```python
from build123d import *

# Parameters (mm, degrees)
SKETCH1_R             = 1.4000000000000001
BOSS_EXTRUDE1_DEPTH   = 8
SKETCH1_R_2           = 1.4000001329680465
BOSS_EXTRUDE1_2_DEPTH = 8
CUT_EXTRUDE1_DEPTH    = 2
BOSS_EXTRUDE2_REACH   = 38.543
FILLET1_R             = 0.3
FILLET2_R             = 0.5
SKETCH4_W             = 3.300000288709998
SKETCH4_H             = 17
BOSS_EXTRUDE3_DEPTH   = 89
FILLET3_R             = 3
FILLET4_R             = 1
FILLET5_R             = 30
FILLET6_R             = 1
FILLET7_R             = 1
SKETCH5_R             = 1.4000008127885915
CUT_EXTRUDE2_DEPTH    = 117.20130403381272


with BuildPart() as part:
    # Sketch1 → Boss-Extrude1 (new body)
    with BuildSketch(Plane.XY):
        Polygon((-3.0301585163921114, 15.386126765608788), (-18.49637259864768, 15.386126765608788), (-25.90000070631504, 14.542589808684392), (-25.90000070631504, 9.120777419209476), (-3.030158516392113, 9.12077741920948), align=None)
        with Locations((-8.999999881867154, 12.49999987202729)):
            Circle(SKETCH1_R, mode=Mode.SUBTRACT)
    extrude(amount=BOSS_EXTRUDE1_DEPTH)


with BuildPart() as body_2:
    # Sketch1 → Boss-Extrude1 2 (new body)
    with BuildSketch(Plane.XY):
        Polygon((-3.0301585163921114, -15.386126765608788), (-3.0301585163921114, -9.12077741920948), (-25.90000070631504, -9.12077741920948), (-25.90000070631504, -14.542589808684392), (-18.496372598647696, -15.386126765608788), align=None)
        with Locations((-8.999999825719202, -12.500000716819214)):
            Circle(SKETCH1_R_2, mode=Mode.SUBTRACT)
    extrude(amount=BOSS_EXTRUDE1_2_DEPTH)


with BuildPart() as cut_extrude1_tool:
    # Sketch2 → Cut-Extrude1 (new body)
    with BuildSketch(Plane.XY.offset(8)):
        Polygon((-5.997778482081098, 12.499999872027288), (-7.498889181974129, 15.099999872027293), (-8.281088680356937, 16.454809144881214), (-9.718911083377371, 16.454809144881214), (-10.501110581760184, 15.099999872027293), (-12.002221281653215, 12.499999872027287), (-10.501110581760186, 9.899999872027289), (-7.498889181974125, 9.899999872027289), align=None)
        Polygon((-7.498889125826173, -9.900000716819214), (-10.501110525612221, -9.900000716819216), (-12.002221225505249, -12.500000716819212), (-10.501110525612223, -15.100000716819206), (-9.468316266504699, -16.88885284735889), (-8.531683384933698, -16.888852847358898), (-7.498889125826177, -15.100000716819206), (-5.997778425933152, -12.500000716819208), align=None)
    extrude(amount=-CUT_EXTRUDE1_DEPTH)


with BuildPart() as part_1:
    add(part.part)

    # Cut-Extrude1: cut by cut_extrude1_tool
    add(cut_extrude1_tool.part, mode=Mode.SUBTRACT)


with BuildPart() as body_2_1:
    add(body_2.part)

    # Cut-Extrude1: cut by cut_extrude1_tool
    add(cut_extrude1_tool.part, mode=Mode.SUBTRACT)

    # Sketch3 → Boss-Extrude2 (add, up to next)
    with BuildSketch(Plane.XZ.offset(-9.12077741920948), mode=Mode.PRIVATE) as boss_extrude2_sk1:
        Polygon((-25.90000070631504, 8), (-25.90000070631504, 2.699999711290002), (-24.255957938355465, 2.6999997112900025), (-12.725226135105776, 8), (-18.496372598647696, 8), align=None)
    boss_extrude2_tool1 = extrude(boss_extrude2_sk1.sketch, amount=BOSS_EXTRUDE2_REACH, mode=Mode.PRIVATE) - body_2_1.part

    add(part_1.part)  # Boss-Extrude2 merges part
    add(boss_extrude2_tool1.solids().sort_by_distance((-21.447611, 9.120777, 6.037334))[0])

    # Fillet1
    fillet1_edges = [body_2_1.edges().sort_by_distance(p)[0] for p in [
        (-10.335915142728517, 15.386126765608788, 7),
        (-7.664084621005797, 15.386126765608788, 7),
        (-7.664084077117004, -15.386126765608788, 7),
        (-10.33591557432139, -15.386126765608788, 7),
    ]]
    fillet(fillet1_edges, radius=FILLET1_R)

    # Fillet2
    fillet2_edges = [body_2_1.edges().sort_by_distance(p)[0] for p in [
        (-12.725226135105776, 0, 8),
    ]]
    fillet(fillet2_edges, radius=FILLET2_R)

    # Sketch4 → Boss-Extrude3 (add)
    with BuildSketch(Plane.ZY.offset(25.90000070631504)):
        with Locations((6.349999855645001, 0)):
            Rectangle(SKETCH4_W, SKETCH4_H)
    extrude(amount=BOSS_EXTRUDE3_DEPTH)

    # Fillet3
    fillet3_edges = [body_2_1.edges().sort_by_distance(p)[0] for p in [
        (-114.90000070631504, 8.5, 6.349999855645001),
        (-114.90000070631504, -8.5, 6.349999855645001),
    ]]
    fillet(fillet3_edges, radius=FILLET3_R)

    # Fillet4
    fillet4_edges = [body_2_1.edges().sort_by_distance(p)[0] for p in [
        (-3.0301585163921114, 15.386126765608788, 4),
        (-3.0301585163921123, 9.12077741920948, 4),
        (-25.90000070631504, 14.542589808684392, 4),
        (-25.90000070631504, 9.120777419209476, 1.349999855645001),
        (-3.0301585163921114, -9.12077741920948, 4),
        (-25.90000070631504, -9.12077741920948, 1.349999855645001),
        (-25.90000070631504, -14.542589808684392, 4),
        (-3.0301585163921114, -15.386126765608788, 4),
    ]]
    fillet(fillet4_edges, radius=FILLET4_R)

    # Fillet5
    fillet5_edges = [body_2_1.edges().sort_by_distance(p)[0] for p in [
        (-18.49637259864768, 15.38612676560879, 4),
        (-18.496372598647696, -15.386126765608788, 4),
    ]]
    fillet(fillet5_edges, radius=FILLET5_R)

    # Fillet6
    fillet6_edges = [body_2_1.edges().sort_by_distance(p)[0] for p in [
        (-14.465079611353577, 9.120777419209478, 0),
        (-22.601074828066285, 14.918454973167087, 0),
        (-3.0301585163921114, 12.253452092409134, 0),
        (-25.90000070631504, 11.885416556829192, 0),
        (-3.323051735205564, 15.093233546795336, 0),
        (-3.3230517352055653, 9.413670638022932, 0),
        (-25.646058085143018, 14.315937356229982, 0),
        (-25.607107487501587, 9.413670638022928, 0),
        (-25.90000070631504, -11.885416556829192, 0),
        (-14.465079611353575, -9.12077741920948, 0),
        (-3.0301585163921114, -12.253452092409134, 0),
        (-10.411503745491025, -15.386126765608788, 0),
        (-3.323051735205564, -9.413670638022932, 0),
        (-3.323051735205564, -15.093233546795336, 0),
        (-25.646058085143018, -14.315937356229977, 0),
        (-25.607107487501587, -9.413670638022932, 0),
        (-22.601074828066285, -14.918454973167087, 0),
        (-18.493632770900625, -15.337876872709488, 0),
        (-10.411503745491025, 15.386126765608788, 0),
        (-18.493632770900625, 15.337876872709492, 0),
    ]]
    fillet(fillet6_edges, radius=FILLET6_R)

    # Fillet7
    fillet7_edges = [body_2_1.edges().sort_by_distance(p)[0] for p in [
        (-114.90000070631504, 1.78e-15, 8),
        (-114.90000070631504, 0, 4.699999711290002),
        (-68.90000070631504, 8.5, 8),
        (-68.90000070631504, -8.5, 8),
        (-114.02132104987469, 7.621320343559643, 8),
        (-114.02132104987469, -7.621320343559643, 8),
        (-68.90000070631504, -8.5, 4.699999711290002),
        (-68.90000070631504, 8.5, 4.699999711290002),
        (-114.02132104987469, 7.621320343559643, 4.699999711290002),
        (-114.02132104987469, -7.621320343559643, 4.699999711290002),
    ]]
    fillet(fillet7_edges, radius=FILLET7_R)

    # Sketch5 → Cut-Extrude2 (cut, through all)
    with BuildSketch(Plane.XY.offset(8)):
        with Locations((-51.80000095537239, -2.0194977255e-07)):
            Circle(SKETCH5_R)
    extrude(amount=-CUT_EXTRUDE2_DEPTH, mode=Mode.SUBTRACT)


solid = body_2_1.part
```
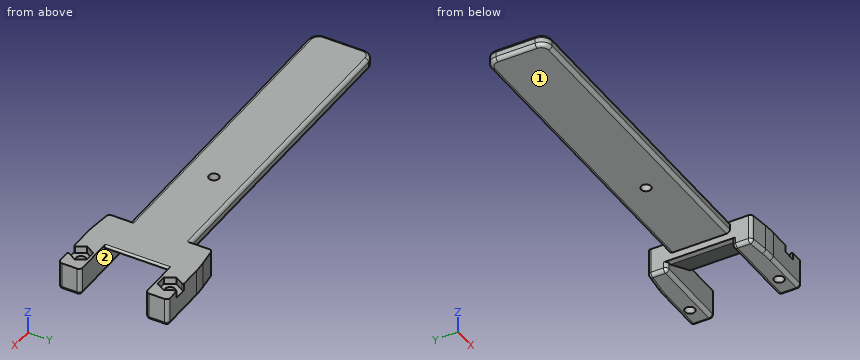
The model under review builds one solid part; all positions refer to its coordinate system, in mm. Face numbers are marked on the shaded views. Round coordinates to 2 decimals unless told otherwise and drop trailing zeros. Order: outer loops, then holes, each group sorted by start corner. A loop starts at its lowest first (then second) coordinate and runs counter-clockwise, first axis right, second up. Notation, with made-up numbers: (-14, 28) -> (-10, 28) arc R6 cw to (-10, 33) -> close; hole circle Ø3 at (12, 0). An arc over 180 degrees is marked (long way). One line per item, written item: value. Start each with the question number.
Q1. Wall thickness on line 1 (Y direction, x = -9, z = 3.5); line 2 (Y direction, x = -51.8, z = 6.1); line 3 (X direction, y = 12.5, z = 4.1): over which ranges is each line inside the solid? List them lowest first.
Q2. Mouldability with a two-part tool opening along Y and no side actions: class the marked faces 1 and 2 as released by +Y, released by -Y, zero draft, split by the parting line, or undercut.
Q3. Take a section at A-A (y = 0). Write out the cut boundary in (x, z), and give its area (3 significant figures).
Q4. Take a section at C-C (x = -70). Write out the cut boundary in (y, z), and give its area (3 significant figures).
Q5. Clearance check with flat-ended pins moving along their axes: pin 1 Ø7.5 at (x, y) = (-70, -0.5) entering from -Z; pin 2 Ø2.5 at (x, y) = (-8, -13) entering from +Z; pin 3 Ø1 at (x, y) = (-69, 8.5) entering from +Z. State where each tip first meets the part, or that it passes through.
Q6. Take a section at B-B (x = -9). Write out the cut boundary in (y, z), and give its area (3 significant figures).
Reported:
1. line 1: y = -15.39 to -13.9, -11.1 to -9.12, 9.12 to 11.1, 13.9 to 15.39
1. line 2: y = -8.5 to -1.4, 1.4 to 8.5
1. line 3: x = -25.9 to -10.4, -7.6 to -3.03
2. face 1: zero draft
2. face 2: undercut
3. outline: (-114.9, 5.7) arc R1 ccw to (-113.9, 4.7) -> (-53.2, 4.7) -> (-53.2, 8) -> (-113.9, 8) arc R1 ccw to (-114.9, 7) -> close; (-50.4, 4.7) -> (-25.9, 4.7) -> (-25.9, 2.7) -> (-24.26, 2.7) -> (-14.8, 7.05) arc R0.5 ccw to (-15.01, 8) -> (-50.4, 8) -> close
3. area: 322 mm2
4. outline: (-8.5, 5.7) arc R1 ccw to (-7.5, 4.7) -> (7.5, 4.7) arc R1 ccw to (8.5, 5.7) -> (8.5, 7) arc R1 ccw to (7.5, 8) -> (-7.5, 8) arc R1 ccw to (-8.5, 7) -> close
4. area: 55.2 mm2
5. pin 1: stops at z = 4.7
5. pin 2: stops at z = 6
5. pin 3: stops at z = 7.87
6. outline: (-15.39, 1) arc R1 ccw to (-14.39, 0) -> (-13.9, 0) -> (-13.9, 6) -> (-15.39, 6) -> close; (-11.1, 0) -> (-10.12, 0) arc R1 ccw to (-9.12, 1) -> (-9.12, 8) -> (-9.9, 8) -> (-9.9, 6) -> (-11.1, 6) -> close; (9.12, 1) arc R1 ccw to (10.12, 0) -> (11.1, 0) -> (11.1, 6) -> (9.9, 6) -> (9.9, 8) -> (9.12, 8) -> close; (13.9, 0) -> (14.39, 0) arc R1 ccw to (15.39, 1) -> (15.39, 6) -> (13.9, 6) -> close
6. area: 43.8 mm2
